```python
from build123d import *

# Parameters (mm, degrees)
SKETCH1_R                      = 35
BOSS_EXTRUDE1_DEPTH            = 1.5
SKETCH4_W                      = 15
SKETCH4_H                      = 21
BOSS_EXTRUDE2_DEPTH            = 5.3
TAP_DRILL_FOR_M2_2X0_45_TAP1_D = 1.75


with BuildPart() as part:
    # Sketch1 → Boss-Extrude1 (new body)
    with BuildSketch(Plane(origin=(0, 0, 0), x_dir=(1, 0, 0), z_dir=(0, 1, 0))):
        with Locations(Location((0, 0, 0), (0, 0, 270))):
            Circle(SKETCH1_R)
    extrude(amount=BOSS_EXTRUDE1_DEPTH)

    # Sketch4 → Boss-Extrude2 (add)
    with BuildSketch(Plane(origin=(0, 1.5, 0), x_dir=(1, 0, 0), z_dir=(0, 1, 0))):
        with Locations((-27.5, 0)):
            Rectangle(SKETCH4_W, SKETCH4_H)
    extrude(amount=BOSS_EXTRUDE2_DEPTH)

    # Tap Drill for M2.2x0.45 Tap1 (through all)
    with Locations(Plane(origin=(-11.5, 1.5, -19.9), x_dir=(0, 0, 1), z_dir=(0, 1, 0))):
        with Locations((0, 0), (12.2, 38.6), (39.8, 0)):
            Hole(TAP_DRILL_FOR_M2_2X0_45_TAP1_D / 2)


solid = part.part
```
Verification items for the finished model (mm, model axes). A direction names the side the tool comes from. Round coordinates to 2 decimals unless told otherwise and drop trailing zeros. Order: outer loops, then holes, each group sorted by start corner. A loop starts at its lowest first (then second) coordinate and runs counter-clockwise, first axis right, second up.
1) Material ranges on line 1 (X direction, y = 5.5, z = 3); line 2 (Y direction, x = 27.5, z = -15); line 3 (X direction, y = 1.25, z = -7.7) (1 decimal), recorded low to high.
Geometry says:
line 1: x = -35 to -20
line 2: y = 0 to 1.5
line 3: x = -34.1 to 26.2, 28 to 34.1
2) Cross-section at C-C, the plane y = 3. Record the cut outline in (x, z).
Geometry says:
outline: (-35, -10.5) - (-20, -10.5) - (-20, 10.5) - (-35, 10.5) - close
3) Depth check by flat-ended pin: pin 1 (3 mm diameter, centred on x = -11.5, z = 19.9, fed in from +Y); pin 2 (2.5 mm diameter, centred on x = -29, y = 3, fed in from +Z); pin 3 (1.5 mm diameter, centred on x = 4.5, y = 1, fed in from +Z). Enter the tip coordinate at first touch or a pass-through.
Geometry says:
pin 1: stops at y = 1.5
pin 2: stops at z = 10.5
pin 3: stops at z = 34.8
4) Tool access check on faces 1 (the flat face through (-28, 4, -10.5)), 2 (the flat face through (-20, 4, 0)), 3 (the flat face through (-34.4, 1.5, 7.9)). Record the directions out of +Z, -Z, +X, -X, +Y, -Y that give a thin tool (end or side, any length) a straight path to the whole face; none if there is none.
Geometry says:
face 1: -Z, +X, -X, +Y
face 2: +Z, -Z, +X, +Y
face 3: +Z, -X, -Y
5) Cross-section at D-D, the plane x = -7. Record the cut outline in (y, z), plus the area to 3 significant figures.
Geometry says:
outline: (0, -34.29) - (1.5, -34.29) - (1.5, 34.29) - (0, 34.29) - close
area: 103 mm2
6) Draft check along Z on faces 4 (the flat face through (0, 0, 0)), 5 (the flat face through (-28, 4, 10.5)), 6 (the cylindrical face through (26.246, 0.74, -7.51)). Enter one of: +Z half, -Z half, draft (parallel to the pull), parting line (faces both ways), or undercut.
Geometry says:
face 4: draft
face 5: +Z half
face 6: undercut
7) Cross-section at A-A, the plane z = 19.9. Record the cut outline in (x, y) (3 decimals), plus the area to 3 significant figures.
Geometry says:
outline: (-28.792, 0) - (-12.375, 0) - (-12.375, 1.5) - (-28.792, 1.5) - close; (-10.625, 0) - (28.792, 0) - (28.792, 1.5) - (-10.625, 1.5) - close
area: 83.8 mm2
8) Cross-section at B-B, the plane z = 7.5. Record the cut outline in (x, y).
Geometry says:
outline: (-35, 1.5) - (-34.19, 1.5) - (-34.19, 0) - (34.19, 0) - (34.19, 1.5) - (-20, 1.5) - (-20, 6.8) - (-35, 6.8) - close
